Model file for the job. Use its own axes, mm. A direction names the side the tool comes from. Coordinates: 2 decimals unless noted, no trailing zeros. Loops run counter-clockwise (first coordinate to the right, second up) from the corner with the lowest first, then second, coordinate; pieces in that order, holes last.
from build123d import *

# Parameters (mm, degrees)
F0_W      = 50
F0_H      = 50
F1_DEPTH  = 50
F3_DEPTH  = 43
F5_DEPTH  = 25
F8_REACH  = 113.7106781187
F10_DEPTH = 35
F12_REACH = 115.9479483752
F13_W     = 20
F13_H     = 10
F14_DEPTH = 30


with BuildPart() as f1:
    # F0 (on Front) → F1 (new body)
    with BuildSketch(Plane.XZ):
        with Locations((-25, 25)):
            Rectangle(F0_W, F0_H)
    extrude(amount=F1_DEPTH)

    # F2 (on face) → F3 (cut)
    with BuildSketch(Plane.XY.offset(50)):
        Polygon((-35, -50), (0, 0), (-50, 0), (-50, -50), align=None)
    extrude(amount=-F3_DEPTH, mode=Mode.SUBTRACT)

    # F4 (on face) → F5 (cut)
    with BuildSketch(Plane.XY.offset(50)):
        Polygon((0, -12.6445109037), (-8.8511576326, -12.6445109037), (-35, -50), (0, -50), align=None)
    extrude(amount=-F5_DEPTH, mode=Mode.SUBTRACT)

    f8_end = Plane(origin=(0, 0, 50), x_dir=(0, -0.8567360565, -0.515755106), z_dir=(0, 0.515755106, -0.8567360565))
    # F6 (on face) → F8 (join, up to a plane its end follows)
    with BuildSketch(Plane.XY.offset(7)):
        Polygon((-50, 0), (-50, -50), (-35, -50), (0, 0), align=None)
    f8_long = extrude(amount=F8_REACH, mode=Mode.PRIVATE)
    add(split(f8_long, bisect_by=f8_end, keep=Keep.TOP, mode=Mode.PRIVATE))

    # F9 (on face) → F10 (cut)
    with BuildSketch(Plane.XY.offset(50)):
        Polygon((-28, -40), (0, 0), (-15, 0), (-43, -40), align=None)
    extrude(amount=-F10_DEPTH, mode=Mode.SUBTRACT)

    f12_end = Plane(origin=(-33.023255814, -47.1760797342, 23.3), x_dir=(-0.5734623444, -0.8192319205, 0), z_dir=(-0.8192319205, 0.5734623444, 0))
    # F11 (on face) → F12 (cut, up to a plane its end follows)
    with BuildSketch(Plane(origin=(-50, 0, 0), x_dir=(0, -1, 0), z_dir=(-1, 0, 0))):
        Polygon((50, 19.9), (0, 50), (50, 7), align=None)
    f12_long = extrude(amount=-F12_REACH, mode=Mode.PRIVATE)
    add(split(f12_long, bisect_by=f12_end, keep=Keep.TOP, mode=Mode.PRIVATE), mode=Mode.SUBTRACT)

    # F13 (on face) → F14 (cut)
    with BuildSketch(Plane.YZ):
        with Locations((-20, 5)):
            Rectangle(F13_W, F13_H)
    extrude(amount=-F14_DEPTH, mode=Mode.SUBTRACT)


solid = f1.part
Q1. Slice it at C-C (y = -4.5). List the corners of the cut face in (x, z), and give its area (3 significant figures).
Answers:
outline: (-50, 0) - (0, 0) - (0, 50) - (-3.15, 50) - (-3.15, 15) - (-18.15, 15) - (-18.15, 46.13) - (-50, 46.13) - close
area: 1,850 mm2
Q2. Drill centre lines: line 1 (Y direction, x = -27.5, z = 3); line 2 (Z direction, x = -17.5, y = -39.5); line 3 (Z direction, x = -26.5, y = -20). Where is each one in solid material? Low to high.
Answers:
line 1: y = -50 to -30, -10 to 0
line 2: z = 0 to 25
line 3: z = 10 to 15
Q3. Slice it at D-D (z = 26). List the corners of the cut face in (x, y), and give its area (3 significant figures).
Answers:
outline: (-50, -27.91) - (-34.53, -27.91) - (-15, 0) - (-50, 0) - close; (-8.85, -12.64) - (0, -12.64) - (0, 0) - close
area: 760 mm2
Q4. Slice it at A-A (x = -39.5). List the corners of the cut face in (y, z).
Answers:
outline: (-50, 0) - (0, 0) - (0, 50) - (-35, 19.9) - (-35, 15) - (-40, 15) - (-40, 15.6) - (-50, 7) - close
Q5. Slice it at B-B (z = 43.5). List the corners of the cut face in (x, y).
Answers:
outline: (-50, -7.56) - (-20.29, -7.56) - (-15, 0) - (-50, 0) - close; (-8.85, -12.64) - (0, -12.64) - (0, 0) - close
Q6. Flat gauge pins, fed straight in: P1, Ø1, axis at x = -39.5, y = -43, coming from the +Z side; P2, Ø10, axis at x = -18, y = -21, coming from the -Z side; P3, Ø6, axis at x = -20.5, y = -33, coming from the +Z side. Where does each tip first touch, or does it go through?
Answers:
P1: stops at z = 13.45
P2: stops at z = 10
P3: stops at z = 25
Q7. Mould opens along Y. For faces 5 (the flat face through (-4, -12.645, 38)), 6 (the flat face through (-30, 0, 25)), 7 (the flat face through (-15, -10, 5)) say: +Y half, -Y half, draft (parallel to the pull), parting line (faces both ways), or undercut.
Answers:
face 5: -Y half
face 6: +Y half
face 7: undercut
Q8. Which spindle directions (+Z, -Z, +X, -X, +Y, -Y) get a long thin tool onto all of the face, cutting with end or side? Do faces 1 (the flat face through (-14, -35, 25)), 2 (the flat face through (-30, -20, 5)), 3 (the flat face through (-3, -9, 50)), 4 (the flat face through (-25.693, -15.276, 28.856)). Say none if no direction does.
Answers:
face 1: +Z, +X, -Y
face 2: -Z, +X
face 3: +Z, +X, -X, +Y, -Y
face 4: +Z
